Can you work these out from the model? Positions are in its coordinate system, mm. A direction names the side the tool comes from. Coordinates: 2 decimals unless noted, no trailing zeros. Write each loop counter-clockwise with the first axis right and the second up, starting at its lowest first coordinate (ties: lowest second). Pieces come first, ordered by that corner, then holes. Notation, with made-up numbers: (80, 24.25) - (125, 24.25) arc R29 cw to (125, 44.25) - close; hole circle Ø7 at (-38, -2). An arc over 180 degrees is marked (long way). Use one line per item in the form item = value. Start each with the question number.
(1) On a 3-axis mill with a long thin cutter (end or side, diameter ignored), from which of +Z, -Z, +X, -X, +Y, -Y can I reach the whole of each face in a straight line? I mean faces 4 (the face through (20.5, 10.4, 0.2)), 5 (the face through (-2.75, 15, 15)), 6 (the face through (2.75, 15, -15)). Say none if no direction works.
(2) Thinking about a two-plate mould opening in Z: for faces 1 (the face through (17.5, 35, -16)), 2 (the face through (13.721, 16.365, 3.634)), 3 (the face through (0.245, -42.634, 5.598)), which applies, pulls with the +Z half, pulls with the -Z half, needs draft (parallel to the pull), parting line crosses it, or undercut?
(3) If we section it at A-A on z = 0: Give the number of separate pieces and of enclosed holes in the cut face, then the cut area to 3 significant figures.
(4) For pin 1 Ø1 at (y, z) = (32.5, 28.5) entering from +X; pin 2 Ø11.5 at (y, z) = (-26.5, 0) entering from +X; pin 3 Ø1.5 at (x, y) = (-4, 5) entering from -Z, each with a flat end and sliding along its axis, tell me the tip position at first contact or that it passes through.
(5) If we section it at C-C on x = 1: Please give me the cut outline in (y, z), then the cut area to 3 significant figures.
(6) If I drill on probe 1 along Y at (x, z) = (0, 0); probe 2 along Y at (x, z) = (5.5, -11); probe 3 along Z at (x, y) = (-15, -1), over which ranges is the centre line in solid material (lowest first)? Write a range as from..to.
(7) If we section it at D-D on x = 7: Please give me the cut outline in (y, z).
```python
from build123d import *

# Parameters (mm, degrees)
CUT_EXTRUDE1_DEPTH      = 74.341666193
CUT_EXTRUDE1_DEPTH_BACK = 74.341666193
SKETCH4_R               = 5
CUT_EXTRUDE2_DEPTH      = 74.341666193
CUT_EXTRUDE2_DEPTH_BACK = 74.341666193
SKETCH5_R               = 10


with BuildPart() as part:
    # Sketch1 → Revolve1 (revolve)
    with BuildSketch(Plane(origin=(0, 0, 0), x_dir=(1, 0, 0), z_dir=(0, 1, 0))):
        Polygon((20.5, 0), (-20.5, 0), (-20.5, 16), (-2.75, 18), (-2.75, 35), (-17.5, 38), (-17.5, 43), (17.5, 43), (17.5, 38), (2.75, 35), (2.75, 18), (20.5, 16), align=None)
    revolve(axis=Axis((20.5, 0, 0), (-1, 0, 0)))

    # Sketch4 → Cut-Extrude1 (cut, two sides: drawn at the far end of the back side and taken through both)
    with BuildSketch(Plane.ZY.offset(20.5).offset(-CUT_EXTRUDE1_DEPTH_BACK)):
        with Locations((0, 26.5)):
            Circle(SKETCH4_R)
        with Locations((26.5, 0)):
            Circle(SKETCH4_R)
        with Locations((0, -26.5)):
            Circle(SKETCH4_R)
        with Locations((-26.5, 0)):
            Circle(SKETCH4_R)
    extrude(amount=CUT_EXTRUDE1_DEPTH + CUT_EXTRUDE1_DEPTH_BACK, mode=Mode.SUBTRACT)

    # Sketch5 → Cut-Extrude2 (cut, two sides: drawn at the far end of the back side and taken through both)
    with BuildSketch(Plane.ZY.offset(20.5).offset(-CUT_EXTRUDE2_DEPTH_BACK)):
        Circle(SKETCH5_R)
    extrude(amount=CUT_EXTRUDE2_DEPTH + CUT_EXTRUDE2_DEPTH_BACK, mode=Mode.SUBTRACT)


solid = part.part
```
Reported:
q1.face_4 = +Z, -Z, +X, +Y, -Y
q1.face_5 = -X
q1.face_6 = +X
q2.face_1 = needs draft
q2.face_2 = undercut
q2.face_3 = parting line crosses it
q3.separate_pieces = 4
q3.enclosed_holes = 0
q3.area = 1,130 mm2
q4.pin_1 = 17.5
q4.pin_2 = 2.75
q4.pin_3 = -42.79
q5.outline = circle Ø86 at (0, 0); hole circle Ø10 at (-26.5, 0); hole circle Ø20 at (0, 0); hole circle Ø10 at (0, -26.5); hole circle Ø10 at (0, 26.5); hole circle Ø10 at (26.5, 0)
q5.area = 5,180 mm2
q6.probe_1 = -43..-31.5, -21.5..-10, 10..21.5, 31.5..43
q6.probe_2 = -41.57..-33.82, -13.85..13.85, 33.82..41.57
q6.probe_3 = -42.99..-37.48, -16.59..-9.95, 9.95..16.59, 37.48..42.99
q7.outline = circle Ø86 at (0, 0); circle Ø35.04 at (0, 0); hole circle Ø71.73 at (0, 0); hole circle Ø20 at (0, 0)
